Verification items for the finished model (mm, model axes). Face numbers are marked on the shaded views. A direction names the side the tool comes from. Round coordinates to 2 decimals unless told otherwise and drop trailing zeros. Loops run counter-clockwise (first coordinate to the right, second up) from the corner with the lowest first, then second, coordinate; pieces in that order, holes last. Notation, with made-up numbers: (-20, 38.25) - (27, 38.25) arc R33 ccw to (27, 69.25) - close; hole circle Ø3 at (70.5, 69.5). An arc over 180 degrees is marked (long way). Use CSV: the item, a comma, the result in double quotes.
```python
from build123d import *

# Parameters (mm, degrees)
BOSS_EXTRUDE2_DEPTH     = 3
SKETCH3_W               = 30
SKETCH3_H               = 8
BOSS_EXTRUDE3_DEPTH     = 2
CUT_EXTRUDE1_DEPTH      = 70.641941386
CUT_EXTRUDE2_DEPTH      = 2
CUT_EXTRUDE2_DEPTH_BACK = 2
SKETCH4_R               = 1.5
CUT_EXTRUDE3_DEPTH      = 2
SKETCH12_R              = 1.5
CUT_EXTRUDE4_DEPTH      = 2


with BuildPart() as part:
    # Sketch1 → Boss-Extrude2 (new body)
    with BuildSketch(Plane(origin=(0, 0, 0), x_dir=(1, 0, 0), z_dir=(0, 1, 0))):
        with BuildLine():
            Line((25, -4), (65, -4))
            ThreePointArc((65, -4), (69, 0), (65, 4))
            Line((65, 4), (25, 4))
            Line((25, 4), (25, -4))
        make_face()
    extrude(amount=BOSS_EXTRUDE2_DEPTH)

    # Sketch3 → Boss-Extrude3 (add)
    with BuildSketch(Plane(origin=(0, 3, 0), x_dir=(1, 0, 0), z_dir=(0, 1, 0))):
        with Locations((40, 0)):
            Rectangle(SKETCH3_W, SKETCH3_H)
    extrude(amount=BOSS_EXTRUDE3_DEPTH)

    # Sketch13 → Cut-Extrude1 (cut, through all)
    with BuildSketch(Plane.XY.offset(4)):
        with BuildLine():
            Line((31.5, 5), (28.5, 5))
            ThreePointArc((28.5, 5), (30, 3.5), (31.5, 5))
        make_face()
    extrude(amount=-CUT_EXTRUDE1_DEPTH, mode=Mode.SUBTRACT)

    # Sketch14 → Cut-Extrude2 (cut, two sides: drawn at the far end of the back side and taken through both)
    with BuildSketch(Plane.XY.offset(-CUT_EXTRUDE2_DEPTH_BACK)):
        with BuildLine():
            Line((27, 5), (33, 5))
            ThreePointArc((33, 5), (30, 2), (27, 5))
        make_face()
    extrude(amount=CUT_EXTRUDE2_DEPTH + CUT_EXTRUDE2_DEPTH_BACK, mode=Mode.SUBTRACT)

    # Sketch4 → Cut-Extrude3 (cut)
    with BuildSketch(Plane(origin=(0, 3, 0), x_dir=(1, 0, 0), z_dir=(0, 1, 0))):
        with Locations(Location((65, 0, 0), (0, 0, 270))):
            Circle(SKETCH4_R)
    extrude(amount=-CUT_EXTRUDE3_DEPTH, mode=Mode.SUBTRACT)

    # Sketch12 → Cut-Extrude4 (cut)
    with BuildSketch(Plane(origin=(0, 5, 0), x_dir=(1, 0, 0), z_dir=(0, 1, 0))):
        with Locations(Location((47, 0, 0), (0, 0, 270))):
            Circle(SKETCH12_R)
    extrude(amount=-CUT_EXTRUDE4_DEPTH, mode=Mode.SUBTRACT)


solid = part.part
```
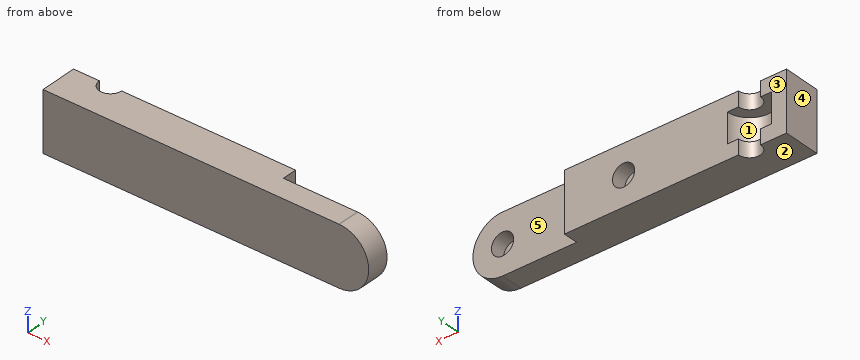
1) Thickness scan on probe 1 along X at (y, z) = (2.5, 0); probe 2 along Z at (x, y) = (31.5, 3.15); probe 3 along Z at (x, y) = (65, 1.9). Record the ranges inside material, lowest first. Write a range as [from, to].
Returned:
probe 1,"x = [25, 28.34], [31.66, 63.5], [66.5, 69]"
probe 2,"z = [-4, -2], [2, 4]"
probe 3,"z = [-4, -1.5], [1.5, 4]"
2) Cross-section at C-C, the plane x = 30. Record the cut outline in (y, z), then the cut area to 3 significant figures.
Returned:
outline,"(0, -4) - (3.5, -4) - (3.5, -2) - (2, -2) - (2, 2) - (3.5, 2) - (3.5, 4) - (0, 4) - close"
area,"22.0 mm²"
3) Access from +Z, -Z, +X, -X, +Y, -Y to the whole of each face (thin tool, end or side, straight path). Record for the marked faces 4 and 5.
Returned:
face 4,"+Z, -Z, -X, +Y, -Y"
face 5,"+Z, -Z, +X, +Y"
4) Cross-section at D-D, the plane x = 61.5. Record the cut outline in (y, z), then the cut area to 3 significant figures.
Returned:
outline,"(0, -4) - (3, -4) - (3, 4) - (0, 4) - close"
area,"24.0 mm²"
5) Mould release check, pull along Z, two halves, no side actions. Record for the marked faces 1, 2 and 3: +Z half, -Z half, draft (parallel to the pull), parting line (faces both ways), or undercut.
Returned:
face 1,"undercut"
face 2,"-Z half"
face 3,"draft"
6) Gauge pin test, flat ends, axial feed: pin 1 Ø1.5 at (x, z) = (65.5, 0.5) entering from +Y; pin 2 Ø1.5 at (x, z) = (46.5, 0) entering from +Y; pin 3 Ø1.6 at (y, z) = (3.5, -1.5) entering from +X. Record the tip position at first contact, or that the pin passes through.
Returned:
pin 1,"stops at y = 1"
pin 2,"stops at y = 3"
pin 3,"stops at x = 68.9"
7) Cross-section at A-A, the plane x = 47. Record the cut outline in (y, z), then the cut area to 3 significant figures.
Returned:
outline,"(0, -4) - (5, -4) - (5, -1.5) - (3, -1.5) - (3, 1.5) - (5, 1.5) - (5, 4) - (0, 4) - close"
area,"34.0 mm²"
8) Cross-section at B-B, the plane z = 0. Record the cut outline in (x, y).
Returned:
outline,"(25, 0) - (69, 0) - (69, 3) - (66.5, 3) - (66.5, 1) - (63.5, 1) - (63.5, 3) - (55, 3) - (55, 5) - (48.5, 5) - (48.5, 3) - (45.5, 3) - (45.5, 5) - (33, 5) arc R3 cw to (27, 5) - (25, 5) - close"
